from build123d import *

# Parameters (mm, degrees)
F1_DEPTH = 19.05
F2_R     = 25.5905
F3_DEPTH = 19.051
F4_SIZE  = 6.35
F5_SIZE  = 4.7625


with BuildPart() as f1:
    # F0 (on Top) → F1 (new body)
    with BuildSketch(Plane.XY):
        with BuildLine():
            Line((47.625, 0), (0, 0))
            Line((0, 0), (0, -94.996))
            Line((0, -94.996), (47.625, -94.996))
            ThreePointArc((47.625, -94.996), (95.123, -47.498), (47.625, 0))
        make_face()
    extrude(amount=F1_DEPTH)

    # F2 (on face) → F3 (cut, through all)
    with BuildSketch(Plane.XY.offset(19.05)):
        with Locations((47.625, -47.498)):
            Circle(F2_R)
    extrude(amount=-F3_DEPTH, mode=Mode.SUBTRACT)

    # F4
    f4_edges = [f1.edges().sort_by_distance(p)[0] for p in [
        (0, 0, 9.525),
        (0, -94.996, 9.525),
        (22.0345, -47.498, 19.05),
        (22.0345, -47.498, 0),
    ]]
    chamfer(f4_edges, length=F4_SIZE)

    # F5
    f5_edges = [f1.edges().sort_by_distance(p)[0] for p in [
        (0, -47.498, 19.05),
        (0, -47.498, 0),
    ]]
    chamfer(f5_edges, length=F5_SIZE)


solid = f1.part
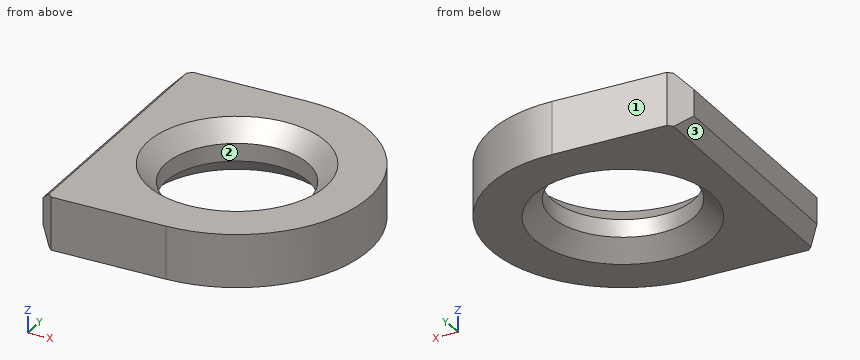
Check sheet for the modelled part. Datum: model origin and axes. Units: mm. Face numbers are marked on the shaded views. Coordinates: 2 decimals unless noted, no trailing zeros. Loops run counter-clockwise (first coordinate to the right, second up) from the corner with the lowest first, then second, coordinate; pieces in that order, holes last. Notation, with made-up numbers: (49.25, 69) -> (70.25, 69) arc R16 ccw to (70.25, 78) -> close; hole circle Ø5 at (82.25, 52). An arc over 180 degrees is marked (long way). Write item = value, one per line. Start each with the question number.
1. Draft check along Y on the marked faces 1, 2 and 3. Enter one of: released by +Y, released by -Y, zero draft, split by the parting line, or undercut.
2. Depth check by flat-ended pin: P1, Ø1.5, axis at y = -73, z = 10.5, coming from the +X side; P2, Ø2, axis at x = 52, z = 11, coming from the +Y side; P3, Ø2, axis at x = 64.5, z = 12.5, coming from the +Y side. Enter the tip coordinate at first touch or a pass-through.
3. Section check B-B on y = -12. Record the cut outline in (x, z), then the cut area to 3 significant figures.
4. Material ranges on line 1 (X direction, y = -49, z = 12.25); line 2 (X direction, y = -36, z = 3); line 3 (Y direction, x = 68, z = 13.75), recorded low to high.
Responses:
q1.face_1 = released by +Y
q1.face_2 = undercut
q1.face_3 = zero draft
q2.P1 = 88.16
q2.P2 = -0.12
q2.P3 = -2.73
q3.outline = (0, 4.76) -> (4.76, 0) -> (79.18, 0) -> (79.18, 19.05) -> (4.76, 19.05) -> (0, 14.29) -> close
q3.area = 1,490 mm2
q4.line_1 = 0 to 22.08, 73.17 to 95.1
q4.line_2 = 1.76 to 21.07, 74.18 to 93.71
q4.line_3 = -90.4 to -64.66, -30.33 to -4.59
